Read the model definition and answer for the solid it produces. Units are mm, in the model's axes. Coordinates: 2 decimals unless noted, no trailing zeros. Order: outer loops, then holes, each group sorted by start corner. A loop starts at its lowest first (then second) coordinate and runs counter-clockwise, first axis right, second up. Notation, with made-up numbers: (17, -10.75) -> (68, -10.75) arc R5 cw to (68, -5.75) -> close; hole circle Ø7 at (58.25, -38). An arc over 180 degrees is marked (long way). Answer as a JSON object with one key per item and string values. Group by question number.
1) Given pin 1 (4.5 mm diameter, centred on x = 1.5, y = 12.73, fed in from +Z), flat-ended and moving along its own axis, determine where the tip first touches the part or whether it passes through.
2) Section A-A on y = 73.69 is taken. Determine the outline of the cut face in (x, z).
3) Determine the mould class of faces 1 (the flat face through (0, 44, 6)), 2 (the flat face through (0, 44, -6)), 3 (the flat face through (0, 87, 0)) for opening direction Z: released by +Z, released by -Z, zero draft, split by the parting line, or undercut.
4) Consider L1, parallel to Y at x = 0, z = 3; L2, parallel to X at y = 73.69, z = 3; L3, parallel to X at y = 59.5, z = -5.5. Determine where each line is inside the solid, lowest interval first.
5) Section B-B on z = 1 is taken. Count the separate pieces of the cut face and the enclosed holes in it, and give its area (3 significant figures).
from build123d import *

# Parameters (mm, degrees)
SKETCH_1_W      = 15
SKETCH_1_H      = 87
SKETCH_1_R      = 1.35
EXTRUDE_1_DEPTH = 12


with BuildPart() as part:
    # 草圖1 → 填料-伸長1 (new body)
    with BuildSketch(Plane(origin=(0, 0, -6), x_dir=(-1, 0, 0), z_dir=(0, 0, -1))):
        with Locations((0, 43.5)):
            Rectangle(SKETCH_1_W, SKETCH_1_H)
        with Locations((-1.5, 22.89)):
            Circle(SKETCH_1_R, mode=Mode.SUBTRACT)
        with Locations((-1.5, 43.21)):
            Circle(SKETCH_1_R, mode=Mode.SUBTRACT)
        with Locations((0, 60.1)):
            Circle(SKETCH_1_R, mode=Mode.SUBTRACT)
        with Locations((0, 6)):
            Circle(SKETCH_1_R, mode=Mode.SUBTRACT)
        with Locations((-1.5, 12.73)):
            Circle(SKETCH_1_R, mode=Mode.SUBTRACT)
        with Locations((-1.5, 33.05)):
            Circle(SKETCH_1_R, mode=Mode.SUBTRACT)
        with Locations((-1.5, 53.37)):
            Circle(SKETCH_1_R, mode=Mode.SUBTRACT)
        with Locations((-1.5, 73.69)):
            Circle(SKETCH_1_R, mode=Mode.SUBTRACT)
    extrude(amount=-EXTRUDE_1_DEPTH)


solid = part.part
Worked answers:
{
 "1": {"pin 1": "stops at z = 6"},
 "2": {"outline": "(-7.5, -6) -> (0.15, -6) -> (0.15, 6) -> (-7.5, 6) -> close; (2.85, -6) -> (7.5, -6) -> (7.5, 6) -> (2.85, 6) -> close"},
 "3": {"face 1": "released by +Z", "face 2": "released by -Z", "face 3": "zero draft"},
 "4": {"L1": "y = 0 to 4.65, 7.35 to 58.75, 61.45 to 87", "L2": "x = -7.5 to 0.15, 2.85 to 7.5", "L3": "x = -7.5 to -1.21, 1.21 to 7.5"},
 "5": {"separate pieces": "1", "enclosed holes": "8", "area": "1,260 mm²"}
}
